Work out the finished part from the listing and answer in its coordinate system (mm). Give positions to 0.01 mm unless a question says otherwise; leave off trailing zeros. Order: outer loops, then holes, each group sorted by start corner. A loop starts at its lowest first (then second) coordinate and runs counter-clockwise, first axis right, second up. Notation, with made-up numbers: (13.25, -13) -> (52.25, -13) arc R23 cw to (52.25, 9) -> close; hole circle Ø10 at (-34.75, 9.5). An arc over 180 degrees is marked (long way). Answer as CSV lines item,"result". Start each with the question number.
1. A cutting plane is placed at B-B (z = 5.08). Give the vertices of the cut face in (x, y).
2. A cutting plane is placed at A-A (x = -50.5). Give the vertices of the cut face in (y, z), then the cut area to 3 significant figures.
3. Flat-ended cylindrical pins translate along their axes: pin 1 (2 mm diameter, centred on y = 9, z = 5, fed in from +X); pin 2 (0.8 mm diameter, centred on y = 8.5, z = 5, fed in from -X). Find the tip coordinate at first contact, or state that the pin passes through.
4. Find the intervals of material crossed by L1, parallel to X at y = 9.5, z = 5.25, in increasing order.
5. A cutting plane is placed at C-C (y = 8.75). Give the vertices of the cut face in (x, z), then the cut area to 3 significant figures.
from build123d import *

# Parameters (mm, degrees)
F0_W     = 114.3
F0_H     = 10.16
F1_DEPTH = 10.16
F3_R     = 1.27
F4_DEPTH = 12.7
F2_R     = 1.27
F5_DEPTH = 12.7


with BuildPart() as f1:
    # F0 (on Top) → F1 (new body)
    with BuildSketch(Plane.XY):
        with Locations((-4.017718, 8.943918)):
            Rectangle(F0_W, F0_H)
    extrude(amount=F1_DEPTH)

    # F3 (on face) → F4 (cut)
    with BuildSketch(Plane.YZ.offset(53.132282)):
        with Locations((8.943918, 5.08)):
            Circle(F3_R)
    extrude(amount=-F4_DEPTH, mode=Mode.SUBTRACT)

    # F2 (on face) → F5 (cut)
    with BuildSketch(Plane(origin=(-61.167718, 0, 0), x_dir=(0, -1, 0), z_dir=(-1, 0, 0))):
        with Locations((-8.943918, 5.08)):
            Circle(F2_R)
    extrude(amount=-F5_DEPTH, mode=Mode.SUBTRACT)


solid = f1.part
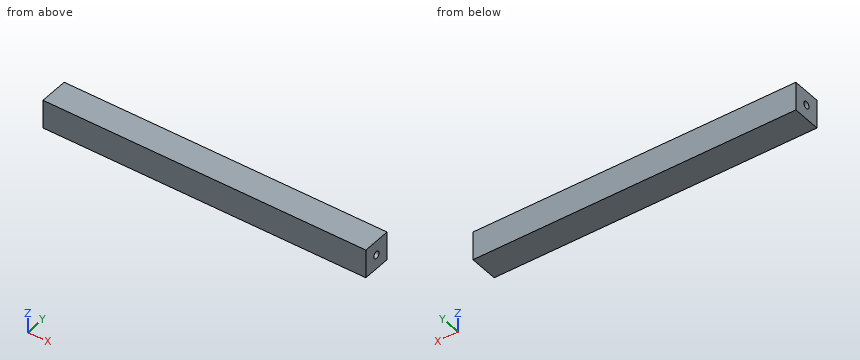
Answer sheet:
1,outline,"(-61.17, 3.86) -> (53.13, 3.86) -> (53.13, 7.67) -> (40.43, 7.67) -> (40.43, 10.21) -> (53.13, 10.21) -> (53.13, 14.02) -> (-61.17, 14.02) -> (-61.17, 10.21) -> (-48.47, 10.21) -> (-48.47, 7.67) -> (-61.17, 7.67) -> close"
2,outline,"(3.86, 0) -> (14.02, 0) -> (14.02, 10.16) -> (3.86, 10.16) -> close; hole circle Ø2.54 at (8.94, 5.08)"
2,area,"98.2 mm^2"
3,pin 1,"stops at x = 40.43"
3,pin 2,"stops at x = -48.47"
4,L1,"x = -48.47 to 40.43"
5,outline,"(-61.17, 0) -> (53.13, 0) -> (53.13, 3.82) -> (40.43, 3.82) -> (40.43, 6.34) -> (53.13, 6.34) -> (53.13, 10.16) -> (-61.17, 10.16) -> (-61.17, 6.34) -> (-48.47, 6.34) -> (-48.47, 3.82) -> (-61.17, 3.82) -> close"
5,area,"1,100 mm^2"
